from build123d import *

# Parameters (mm, degrees)
SKETCH_1_R          = 5
EXTRUDE_1_DEPTH     = 2
SKETCH_2_R          = 3.5
EXTRUDE_2_DEPTH     = 9
SKETCH_3_R          = 2.5
CUT_EXTRUDE_1_DEPTH = 12


with BuildPart() as part:
    # Эскиз1 → Бобышка-Вытянуть1 (new body)
    with BuildSketch(Plane(origin=(0, 0, 0), x_dir=(1, 0, 0), z_dir=(0, 1, 0))):
        Circle(SKETCH_1_R)
    extrude(amount=EXTRUDE_1_DEPTH)

    # Эскиз2 → Бобышка-Вытянуть2 (add)
    with BuildSketch(Plane(origin=(0, 2, 0), x_dir=(1, 0, 0), z_dir=(0, 1, 0))):
        Circle(SKETCH_2_R)
    extrude(amount=EXTRUDE_2_DEPTH)

    # Эскиз3 → Вырез-Вытянуть1 (cut, through all)
    with BuildSketch(Plane(origin=(0, 11, 0), x_dir=(1, 0, 0), z_dir=(0, 1, 0))):
        Circle(SKETCH_3_R)
    extrude(amount=-CUT_EXTRUDE_1_DEPTH, mode=Mode.SUBTRACT)


solid = part.part
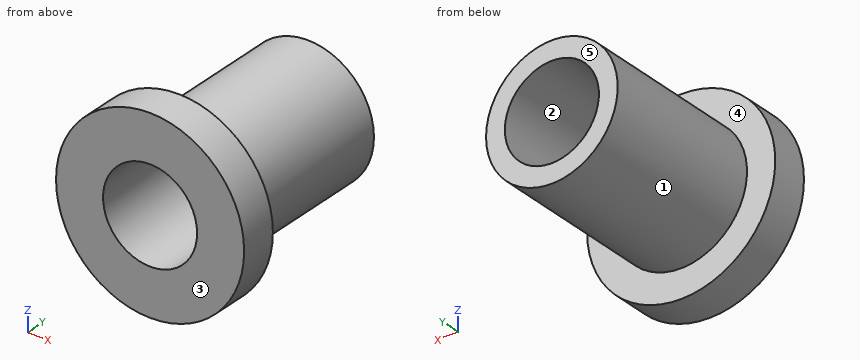
Could you check a few things on this model? Use its own coordinates, in mm. Face numbers are marked on the shaded views. A direction names the side the tool comes from. Give positions to 0.01 mm unless a question says otherwise; leave off trailing zeros. Order: outer loops, then holes, each group sorted by start corner. A loop starts at its lowest first (then second) coordinate and runs counter-clockwise, first axis right, second up. Notation, with made-up numbers: (75, 21) - (94, 21) arc R14 cw to (94, 47) - close; hole circle Ø3 at (65, 0). An arc over 180 degrees is marked (long way). One line per question, with ' | ' between items. Start each with the question number.
Item 1: I want a section at C-C on y = 2.5. Write out the boundary of the cut face in (x, z), then the cut area to 3 significant figures.
Item 2: I need wall thicknesses on probe 1 along Z at (x, y) = (0, 8.75); probe 2 along Y at (x, z) = (-2, -4). Which ranges of each line are inside material? Lowest first, please. Write a range as [from, to].
Item 3: Thinking about a two-plate mould opening in X: for the marked faces 1, 2 and 3, which applies, pulls with the +X half, pulls with the -X half, needs draft (parallel to the pull), parting line crosses it, or undercut?
Item 4: I want a section at B-B on x = 0. Write out the boundary of the cut face in (y, z).
Item 5: I'm going to push flat-ended pins straight in: pin 1 Ø1.5 at (x, y) = (-3, 2.5) entering from +Z; pin 2 Ø1 at (y, z) = (4, -2) entering from -X; pin 3 Ø2 at (y, z) = (7.5, 0.5) entering from +X. Where does each tip first touch, or does it pass through?
Item 6: I want a section at A-A on z = 0. Write out the boundary of the cut face in (x, y).
Item 7: For the marked faces 4 and 5, which set-ups out of +Z, -Z, +X, -X, +Y, -Y let a thin tool reach every point of the face, with its end or its side?
Item 8: I want a section at D-D on x = -3. Write out the boundary of the cut face in (y, z), then the cut area to 4 significant figures.
Verdict:
1) outline: circle Ø7 at (0, 0); hole circle Ø5 at (0, 0) | area: 18.8 mm^2
2) probe 1: [-3.5, -2.5], [2.5, 3.5] | probe 2: [0, 2]
3) face 1: parting line crosses it | face 2: undercut | face 3: needs draft
4) outline: (0, -5) - (2, -5) - (2, -3.5) - (11, -3.5) - (11, -2.5) - (0, -2.5) - close; (0, 2.5) - (11, 2.5) - (11, 3.5) - (2, 3.5) - (2, 5) - (0, 5) - close
5) pin 1: z = 4.36 | pin 2: x = -3.16 | pin 3: x = 3.5
6) outline: (-5, 0) - (-2.5, 0) - (-2.5, 11) - (-3.5, 11) - (-3.5, 2) - (-5, 2) - close; (2.5, 0) - (5, 0) - (5, 2) - (3.5, 2) - (3.5, 11) - (2.5, 11) - close
7) face 4: +Y | face 5: +Z, -Z, +X, -X, +Y
8) outline: (0, -4) - (2, -4) - (2, -1.8) - (11, -1.8) - (11, 1.8) - (2, 1.8) - (2, 4) - (0, 4) - close | area: 48.45 mm^2
